For this review, use the dimensioned drawing (mm, ordinates from the lowest corner) and the shaded views. A direction names the side the tool comes from. Round coordinates to 2 decimals unless told otherwise and drop trailing zeros. Loops run counter-clockwise (first coordinate to the right, second up) from the corner with the lowest first, then second, coordinate; pieces in that order, holes last. Notation, with made-up numbers: (22, 50) -> (64, 50) arc R5 ccw to (64, 56) -> close; hole circle Ø1 at (33, 4). An arc over 180 degrees is marked (long way). Use one line per item in the form item = value. Start each with the question number.
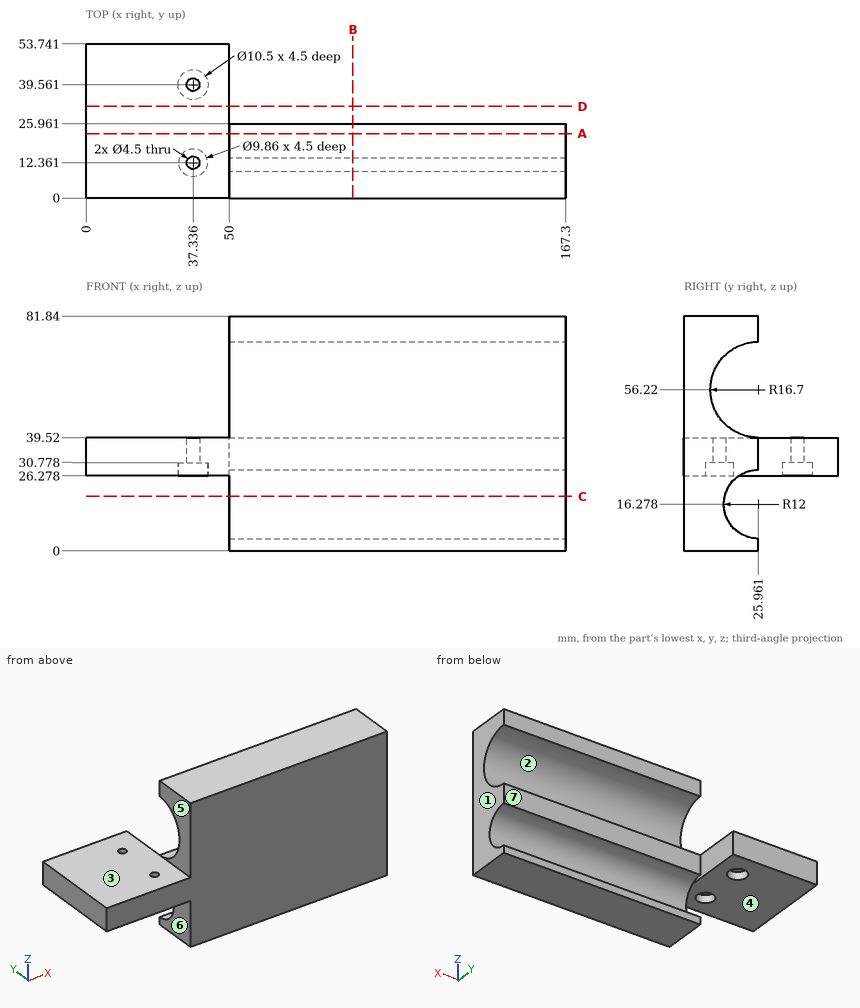
Item 1: Machinability: for the marked faces 5, 6 and 7, which of the approach directions +Z, -Z, +X, -X, +Y, -Y give a long, thin tool a straight path to every point of the face, cutting with its end or side? Answer none if there is none.
Item 2: Take a section at A-A on y = 22.5. Give the boundary of the cut face in (x, z), plus the area to 3 significant figures.
Item 3: Draft analysis for pull direction Z (two halves, no side actions). For the marked faces 1, 2, 3 and 4, state which applies: +Z half, -Z half, draft (parallel to the pull), parting line (faces both ways), or undercut.
Item 4: For P1, Ø4, axis at x = 37.34, y = 39.56, coming from the +Z side; P2, Ø8, axis at x = 37.34, y = 12.36, coming from the +Z side; P3, Ø8, axis at x = 38, y = 14, coming from the -Z side; P4, Ø5.5, axis at x = 99, z = 36, coming from the +Y side, all flat-tipped, find the tip position at first contact; note any pin that passes through.
Item 5: Take a section at D-D on y = 32. Give the boundary of the cut face in (x, z).
Item 6: Take a section at C-C on z = 19. Give the boundary of the cut face in (x, y), plus the area to 3 significant figures.
Item 7: Take a section at B-B on x = 93. Give the boundary of the cut face in (y, z), plus the area to 3 significant figures.
Item 8: Wall thickness on line 1 (X direction, y = 51, z = 27); line 2 (Z direction, x = 49, y = 26); line 3 (X direction, y = 4.5, z = 75.5): over which ranges is each line inside the solid? List them lowest first.
Results:
q1.face_5 = +Z, -X, +Y, -Y
q1.face_6 = -Z, -X, +Y, -Y
q1.face_7 = +Z, -Z, +X, +Y
q2.outline = (0, 26.28) -> (50, 26.28) -> (50, 27.77) -> (167.3, 27.77) -> (167.3, 39.88) -> (50, 39.88) -> (50, 39.52) -> (0, 39.52) -> close; (50, 0) -> (167.3, 0) -> (167.3, 4.79) -> (50, 4.79) -> close; (50, 72.56) -> (167.3, 72.56) -> (167.3, 81.84) -> (50, 81.84) -> close
q2.area = 3,730 mm2
q3.face_1 = draft
q3.face_2 = undercut
q3.face_3 = +Z half
q3.face_4 = -Z half
q4.P1 = through
q4.P2 = 39.52
q4.P3 = 26.28
q4.P4 = 25.96
q5.outline = (0, 26.28) -> (50, 26.28) -> (50, 39.52) -> (0, 39.52) -> close
q6.outline = (50, 0) -> (167.3, 0) -> (167.3, 14.27) -> (50, 14.27) -> close
q6.area = 1,670 mm2
q7.outline = (0, 0) -> (25.96, 0) -> (25.96, 4.28) arc R12 cw to (25.96, 28.28) -> (25.96, 39.52) arc R16.7 cw to (25.96, 72.92) -> (25.96, 81.84) -> (0, 81.84) -> close
q7.area = 1,460 mm2
q8.line_1 = 0 to 50
q8.line_2 = 26.28 to 39.52
q8.line_3 = 50 to 167.3
